Autodesk Fusion 360 part; units mm, degrees
sketch "草图1" plane through (0, 0, 0) normal (0, 1, 0) x (1, 0, 0)
  circle A0 centre (0, 0) radius 24.125
  circle A1 centre (0, 0) radius 29.375
  dimension "d1" = 48.25
  dimension "d2" = 58.75
extrude "拉伸1" add sketch "草图1" along normal blind 0.8 makes body 1
sketch "草图2" plane through (0, 0, 0) normal (0, -1, 0) x (1, 0, 0)
  circle A0 centre (0, 0) radius 24.125
  circle A1 centre (0, 0) radius 29.375
  circle A2 centre (0, 0) radius 43
  line L0 (2.4024, -17.839) -> (16.6502, 6.839)
  line L1 (-16.6502, 6.839) -> (-2.4024, -17.839)
  arc A3 (-14.2478, 11) -> (-16.6502, 6.839) centre (0, 0) ccw
  line L2 (14.2478, 11) -> (-14.2478, 11)
  arc A4 (16.6502, 6.839) -> (14.2478, 11) centre (0, 0) ccw
  arc A5 (-2.4024, -17.839) -> (2.4024, -17.839) centre (0, 0) ccw
  dimension "d5" = 86
extrude "拉伸2" add sketch "草图2" along normal blind 2 separate body contours A2 makes body 2
extrude "拉伸3" add sketch "草图2" along normal blind 1 contours A0 | A1 bodies 1 2
extrude "拉伸4" add 1 faces at (-15.1728, -1, -7.9151) along direction (0, -1, 0) up to surface (1 mm away) on bodies 1 bodies 1
sketch "草图3" plane through (0, -2, 0) normal (0, -1, 0) x (1, 0, 0)
  line L0 (16.6502, 6.839) -> (2.4024, -17.839)
  arc A0 (-2.4024, -17.839) -> (2.4024, -17.839) centre (0, 0) ccw
  line L1 (-2.4024, -17.839) -> (-16.6502, 6.839)
  arc A1 (-14.2478, 11) -> (-16.6502, 6.839) centre (0, 0) ccw
  line L2 (-14.2478, 11) -> (14.2478, 11)
  arc A2 (16.6502, 6.839) -> (14.2478, 11) centre (0, 0) ccw
  circle A3 centre (0, 0) radius 43
  circle A4 centre (0, 0) radius 29.5
  circle A5 centre (0, 0) radius 24
  dimension "d12" = 59
  dimension "d13" = 48
extrude "拉伸5" cut sketch "草图3" against normal blind 1 contours A4 bodies 1
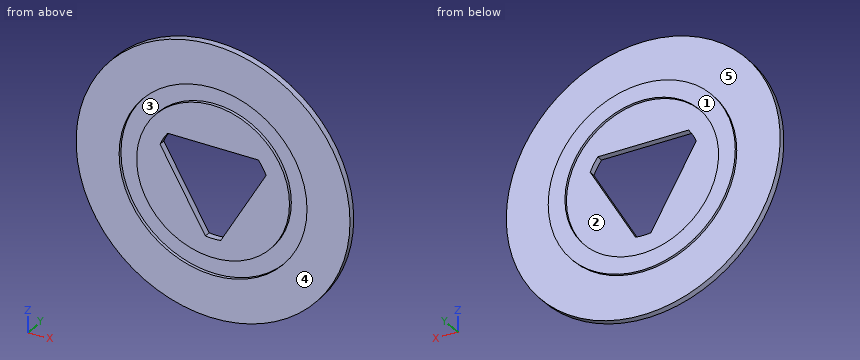
The listing builds one solid part. Answer for the finished solid, in the listing's coordinates (mm). Face numbers are marked on the shaded views. A direction names the side the tool comes from. Give positions to 0.01 mm unless a question says otherwise; leave off trailing zeros. Order: outer loops, then holes, each group sorted by start corner. A loop starts at its lowest first (then second) coordinate and runs counter-clockwise, first axis right, second up. Notation, with made-up numbers: (40, 44.5) -> (55, 44.5) arc R21 ccw to (55, 65.5) -> close; hole circle Ø1 at (-32, 23). An arc over 180 degrees is marked (long way). Put each result on its own line as item: value.
Item 1: A cutting plane is placed at B-B on x = 0. Give the vertices of the cut face in (y, z) (3 decimals).
Established:
outline: (-2, -43) -> (0, -43) -> (0, -29.375) -> (0.8, -29.375) -> (0.8, -24.125) -> (0, -24.125) -> (0, -18) -> (-2, -18) -> (-2, -24) -> (-1, -24) -> (-1, -29.5) -> (-2, -29.5) -> close; (-2, 11) -> (0, 11) -> (0, 24.125) -> (0.8, 24.125) -> (0.8, 29.375) -> (0, 29.375) -> (0, 43) -> (-2, 43) -> (-2, 29.5) -> (-1, 29.5) -> (-1, 24) -> (-2, 24) -> close
Item 2: Straight lines are drawn through the part: line 1 (Z direction, x = 0, y = -1.5); line 2 (Z direction, x = 0, y = 0.55) (3 decimals); line 3 (Z direction, x = 2, y = -1.5). For each, find the intervals that lie inside material, in ascending order.
Established:
line 1: z = -43 to -29.5, -24 to -18, 11 to 24, 29.5 to 43
line 2: z = -29.375 to -24.125, 24.125 to 29.375
line 3: z = -42.95 to -29.43, -23.92 to -17.89, 11 to 23.92, 29.43 to 42.95
Item 3: A cutting plane is placed at D-D on x = -28. Give the vertices of the cut face in (y, z).
Established:
outline: (-2, -32.63) -> (0, -32.63) -> (0, -8.88) -> (0.8, -8.88) -> (0.8, 8.88) -> (0, 8.88) -> (0, 32.63) -> (-2, 32.63) -> (-2, 9.29) -> (-1, 9.29) -> (-1, -9.29) -> (-2, -9.29) -> close
Item 4: Given P1, Ø1, axis at x = -23.5, y = -0.5, coming from the -Z side; P2, Ø1, axis at y = 0, z = 17, coming from the +X side; P3, Ø17.5, axis at x = 4.5, z = -7, coming from the -Y side; P4, Ø14.5, axis at x = 2, z = -9, coming from the +Y side, each flat-ended and moving along its own axis, determine where each tip first touches the part or whether it passes through.
Established:
P1: stops at z = -36.33
P2: stops at x = 39.71
P3: stops at y = -2
P4: stops at y = 0
Item 5: A cutting plane is placed at C-C on z = 0. Give the vertices of the cut face in (x, y) (3 decimals), plus the area to 3 significant figures.
Established:
outline: (-43, -2) -> (-29.5, -2) -> (-29.5, -1) -> (-24, -1) -> (-24, -2) -> (-12.702, -2) -> (-12.702, 0) -> (-24.125, 0) -> (-24.125, 0.8) -> (-29.375, 0.8) -> (-29.375, 0) -> (-43, 0) -> close; (12.702, -2) -> (24, -2) -> (24, -1) -> (29.5, -1) -> (29.5, -2) -> (43, -2) -> (43, 0) -> (29.375, 0) -> (29.375, 0.8) -> (24.125, 0.8) -> (24.125, 0) -> (12.702, 0) -> close
area: 119 mm^2
Item 6: For a pull along Z with two mould halves and no side action, classify the marked faces 1, 2 and 3 as released by +Z, released by -Z, zero draft, split by the parting line, or undercut.
Established:
face 1: zero draft
face 2: undercut
face 3: undercut
Item 7: For the marked faces 4 and 5, determine the directions among +Z, -Z, +X, -X, +Y, -Y from which every point of the face is accessible in a straight line to the end or side of a thin tool.
Established:
face 4: +Z, -Z, +X, -X, -Y
face 5: +Y
Item 8: A cutting plane is placed at A-A on y = -1.45. Give the vertices of the cut face in (x, z).
Established:
outline: circle Ø86 at (0, 0); circle Ø48 at (0, 0); hole circle Ø59 at (0, 0); hole (-16.65, 6.84) -> (-2.4, -17.84) arc R18 ccw to (2.4, -17.84) -> (16.65, 6.84) arc R18 ccw to (14.25, 11) -> (-14.25, 11) arc R18 ccw to start
